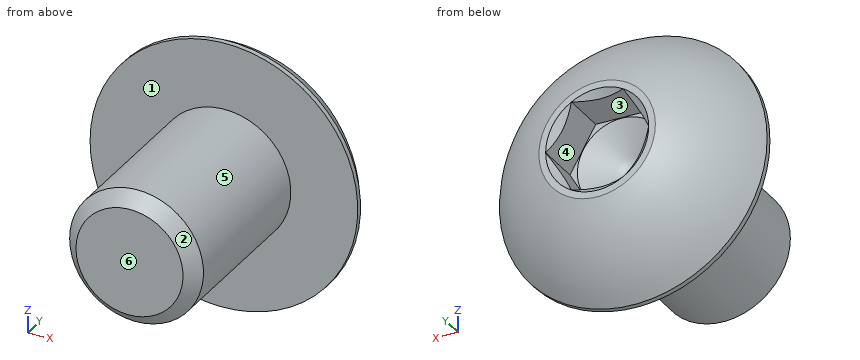
```python
from build123d import *

# Parameters (mm, degrees)
SCHNITT_LINEAR_AUSTRAGEN1_DEPTH = 2.0625


with BuildPart() as part:
    # Skizze1 → Rotation1 (revolve)
    with BuildSketch(Plane(origin=(0, 0, 0), x_dir=(1, 0, 0), z_dir=(0, 0, -1)), mode=Mode.PRIVATE) as rotation1_sk:
        with BuildLine():
            Line((0, 11.3), (2.4, 11.3))
            Line((2.4, 11.3), (3, 10.7))
            Line((3, 10.7), (3, 3.3))
            Line((3, 3.3), (6, 3.3))
            Line((6, 3.3), (6, 3.06135))
            ThreePointArc((6, 3.06135), (4.568743009, 1.238234699), (2.609401077, 0))
            Line((2.609401077, 0), (2.309401077, 0))
            Line((2.309401077, 0), (1.98, 0.329401077))
            Line((1.98, 0.329401077), (1.98, 2.0625))
            Line((1.98, 2.0625), (0, 3.252204026))
            Line((0, 3.252204026), (0, 11.3))
        make_face()
    revolve(rotation1_sk.sketch.rotate(Axis((0, 0, 0), (0, -1, 0)), 180), axis=Axis((0, 0, 0), (0, -1, 0)))  # turned: the seam where the file's is

    # Skizze2 → Schnitt-Linear austragen1 (cut)
    with BuildSketch(Plane(origin=(1.973616694, 0, -1.468825329), x_dir=(-1, 0, 0), z_dir=(0, 1, 0))):
        Polygon((0.818916155, -0.531174671), (3.128317232, -0.531174671), (4.28301777, 1.468825329), (3.128317232, 3.468825329), (0.818916155, 3.468825329), (-0.335784383, 1.468825329), align=None)
    extrude(amount=-SCHNITT_LINEAR_AUSTRAGEN1_DEPTH, mode=Mode.SUBTRACT)


solid = part.part
```
The model under review builds one solid part; all positions refer to its coordinate system, in mm. Face numbers are marked on the shaded views. A direction names the side the tool comes from. Coordinates: 2 decimals unless noted, no trailing zeros. Order: outer loops, then holes, each group sorted by start corner. A loop starts at its lowest first (then second) coordinate and runs counter-clockwise, first axis right, second up. Notation, with made-up numbers: (42, 14) -> (51, 14) arc R33 ccw to (51, 46) -> close; hole circle Ø10 at (30, 24.25). An arc over 180 degrees is marked (long way). Answer in a Markdown table with one row per item. Add a question column.
Item 1: We need section A-A on y = -6.25. Write out the cut boundary in (x, z).
Item 2: To check wall thickness, follow probe 1 along X at (y, z) = (-1.75, -1.25); probe 2 along Y at (x, z) = (-4.25, 0.5); probe 3 along Y at (x, z) = (5, -2.5). State the ranges of each line that lie inside material, in increasing order.
Item 3: Clearance check with flat-ended pins moving along their axes: pin 1 (1 mm diameter, centred on y = -1.5, z = -1, fed in from +X); pin 2 (1.5 mm diameter, centred on y = -9.5, z = -3.5, fed in from +X); pin 3 (2.5 mm diameter, centred on x = 0, y = -0.5, fed in from -Z). State where each tip first meets the part, or that it passes through.
Item 4: Mouldability with a two-part tool opening along X and no side actions: class the marked faces 1, 2 and 3 as +X half, -X half, draft (parallel to the pull), parting line (faces both ways), or undercut.
Item 5: Machinability: for the marked faces 4, 5 and 6, which of the approach directions +Z, -Z, +X, -X, +Y, -Y give a long, thin tool a straight path to every point of the face, cutting with its end or side? Answer none if there is none.
Item 6: We need section B-B on x = -3.75. Write out the cut boundary in (y, z), plus the area to 3 significant figures.
Final values:
| question | item | result |
|---|---|---|
| 1 | outline | circle Ø6 at (0, 0) |
| 2 | probe 1 | x = -4.92 to -1.59, 1.59 to 4.92 |
| 2 | probe 2 | y = -3.3 to -0.99 |
| 2 | probe 3 | y = -3.3 to -2.4 |
| 3 | pin 1 | stops at x = 5.21 |
| 3 | pin 2 | stops at x = 1.2 |
| 3 | pin 3 | stops at z = -5.08 |
| 4 | face 1 | draft |
| 4 | face 2 | parting line |
| 4 | face 3 | undercut |
| 5 | face 4 | +Y |
| 5 | face 5 | -Y |
| 5 | face 6 | +Z, -Z, +X, -X, -Y |
| 6 | outline | (-3.3, -4.68) -> (-3.06, -4.68) arc R5.69 ccw to (-3.06, 4.68) -> (-3.3, 4.68) -> close |
| 6 | area | 18.4 mm2 |
